Read the model definition and answer for the solid it produces. Units are mm, in the model's axes. Give positions to 0.01 mm unless a question says otherwise; leave off trailing zeros. Put each result on its own line as item: value. Start each with the question number.
1. A cutting plane is placed at A-A, the plane y = 0. Count the separate pieces of the cut face and the enclosed holes in it, plus the area to 3 significant figures.
2. For a pull along X with two mould halves and no side action, classify faces 1 (the flat face through (77.5, 2, 2)), 2 (the cylindrical face through (48.81, 0.38, 1.48)), 3 (the flat face through (-77.5, 2, 2)) as released by +X, released by -X, zero draft, split by the parting line, or undercut.
3. Given pin 1 Ø0.5 at (x, z) = (52, 2) entering from +Y, flat-ended and moving along its own axis, determine where the tip first touches the part or whether it passes through.
4. Consider L1, parallel to Y at x = -50, z = 1.2; L2, parallel to Y at x = 24, z = 1.75. Determine where each line is inside the solid, lowest interval first. Write a range as from..to.
```python
from build123d import *

# Parameters (mm, degrees)
SKETCH_1_W             = 155
SKETCH_1_H             = 9
EXTRUDE_1_DEPTH        = 3
SKETCH_3_W             = 155
SKETCH_3_H             = 3
EXTRUDE_2_DEPTH        = 4.25
EXTRUDE_3_DEPTH        = 3
M3X0_5_1_D             = 2.5
PATTERN_LINEAR_1_COUNT = 49
PATTERN_LINEAR_1_PITCH = 3.141592654
PATTERN_LINEAR_2_COUNT = 8
PATTERN_LINEAR_2_PITCH = 20


with BuildPart() as part:
    # 草圖1 → 填料-伸長1 (new body)
    with BuildSketch(Plane.XY):
        Rectangle(SKETCH_1_W, SKETCH_1_H)
    extrude(amount=EXTRUDE_1_DEPTH)

    # 草圖3 → 填料-伸長2 (add)
    with BuildSketch(Plane(origin=(0, 4.5, 0), x_dir=(1, 0, 0), z_dir=(0, 1, 0))):
        with Locations((0, -1.5)):
            Rectangle(SKETCH_3_W, SKETCH_3_H)
    extrude(amount=EXTRUDE_2_DEPTH)

    # 草圖4 → 填料-伸長3 (add, through all)
    with BuildSketch(Plane.XY):
        Polygon((-76.5, 8.75), (-74.019278088, 8.75), (-74.838211115, 11), (-75.681066973, 11), align=None)
    extrude_3 = extrude(amount=EXTRUDE_3_DEPTH)

    # M3x0.5 螺紋孔1 (through all)
    with Locations(Plane.XY.offset(3)):
        with Locations((-70, 0)):
            m3x0_5_1 = Hole(M3X0_5_1_D / 2)

    # 直線複製排列1: 填料-伸長3 ×49
    with Locations(*[(i * PATTERN_LINEAR_1_PITCH, 0, 0) for i in range(1, PATTERN_LINEAR_1_COUNT)]):
        add(extrude_3)

    # 直線複製排列2: M3x0.5 螺紋孔1 ×8
    with Locations(*[(i * PATTERN_LINEAR_2_PITCH, 0, 0) for i in range(1, PATTERN_LINEAR_2_COUNT)]):
        add(m3x0_5_1, mode=Mode.SUBTRACT)


solid = part.part
```
Return value:
1. separate pieces: 9
1. enclosed holes: 0
1. area: 405 mm2
2. face 1: released by +X
2. face 2: undercut
2. face 3: released by -X
3. pin 1: stops at y = 8.75
4. L1: y = -4.5..-1.25, 1.25..11
4. L2: y = -4.5..8.75
